```python
from build123d import *

# Parameters (mm, degrees)
SALIENTE_EXTRUIR1_DEPTH = 4
CROQUIS2_R              = 3
CORTAR_EXTRUIR1_DEPTH   = 4
CROQUIS3_R              = 3
CORTAR_EXTRUIR2_DEPTH   = 4
CROQUIS4_R              = 3
CORTAR_EXTRUIR3_DEPTH   = 4


with BuildPart() as part:
    # Croquis1 → Saliente-Extruir1 (new body)
    with BuildSketch(Plane(origin=(0, 0, 0), x_dir=(1, 0, 0), z_dir=(0, 1, 0))):
        Polygon((-82, -35), (-82, -50), (82, -50), (82, -35), (106, -35), (106, 35), (82, 35), (82, 50), (-82, 50), (-82, 35), (-106, 35), (-106, -35), align=None)
    extrude(amount=SALIENTE_EXTRUIR1_DEPTH)

    # Croquis2 → Cortar-Extruir1 (cut)
    with BuildSketch(Plane(origin=(0, 4, 0), x_dir=(1, 0, 0), z_dir=(0, 1, 0))):
        with Locations(Location((-96, 0, 0), (0, 0, 270))):
            Circle(CROQUIS2_R)
        with Locations(Location((-96, 15, 0), (0, 0, 270))):
            Circle(CROQUIS2_R)
        with Locations(Location((-96, -15, 0), (0, 0, 270))):
            Circle(CROQUIS2_R)
    extrude(amount=-CORTAR_EXTRUIR1_DEPTH, mode=Mode.SUBTRACT)

    # Croquis3 → Cortar-Extruir2 (cut)
    with BuildSketch(Plane(origin=(0, 4, 0), x_dir=(1, 0, 0), z_dir=(0, 1, 0))):
        with Locations(Location((96, 15, 0), (0, 0, 270))):
            Circle(CROQUIS3_R)
        with Locations(Location((96, -15, 0), (0, 0, 270))):
            Circle(CROQUIS3_R)
        with Locations(Location((96, 0, 0), (0, 0, 270))):
            Circle(CROQUIS3_R)
    extrude(amount=-CORTAR_EXTRUIR2_DEPTH, mode=Mode.SUBTRACT)

    # Croquis4 → Cortar-Extruir3 (cut)
    with BuildSketch(Plane(origin=(0, 4, 0), x_dir=(1, 0, 0), z_dir=(0, 1, 0))):
        with Locations(Location((0, 25, 0), (0, 0, 270))):
            Circle(CROQUIS4_R)
        with Locations(Location((50, 0, 0), (0, 0, 270))):
            Circle(CROQUIS4_R)
        with Locations(Location((0, -25, 0), (0, 0, 270))):
            Circle(CROQUIS4_R)
        with Locations(Location((-50, 0, 0), (0, 0, 270))):
            Circle(CROQUIS4_R)
        with Locations(Location((0, 0, 0), (0, 0, 270))):
            Circle(CROQUIS4_R)
    extrude(amount=-CORTAR_EXTRUIR3_DEPTH, mode=Mode.SUBTRACT)


solid = part.part
```
CAD build for the part. Positions are in the model's coordinates, mm. A direction names the side the tool comes from. Coordinates: 2 decimals unless noted, no trailing zeros. Write each loop counter-clockwise with the first axis right and the second up, starting at its lowest first coordinate (ties: lowest second). Pieces come first, ordered by that corner, then holes. Notation, with made-up numbers: (-17, 67) -> (12, 67) arc R18 cw to (12, 101) -> close; hole circle Ø8 at (-1, 23.5). An arc over 180 degrees is marked (long way). Use CSV: the item, a comma, the result in double quotes. Start each with the question number.
Item 1: Drop flat-ended pins along their axis: P1, Ø7, axis at x = -50, z = 0, coming from the +Y side; P2, Ø1.2, axis at x = -97, y = 1.5, coming from the +Z side; P3, Ø1.2, axis at y = 3, z = -39, coming from the +X side; P4, Ø1.5, axis at y = 0.5, z = -38, coming from the -X side. Give the stop position or say it passes through.
Item 2: Wall check: probe 1 along X at (y, z) = (1.95, 0); probe 2 along X at (y, z) = (1.6, -15); probe 3 along Z at (x, y) = (-90, 0.3). Give the ranges that are in metal, low to high.
Item 3: Band-saw the part on A-A, the plane x = -50. Write the cut outline in (y, z).
Item 4: Tool access for faces 1 (the flat face through (82, 2, -42)), 2 (the flat face through (-82, 2, -43)), 3 (the flat face through (-94, 2, 35)), 4 (the flat face through (94, 2, 35)): list every direction of +Z, -Z, +X, -X, +Y, -Y with a clear straight run to the whole face (end or side of a thin tool).
Item 5: Band-saw the part on C-C, the plane y = 1. Give the number of separate pieces and of enclosed holes in the cut face, plus the area to 3 significant figures.
Item 6: Band-saw the part on B-B, the plane z = -15. Write the cut outline in (x, y), plus the area to 3 significant figures.
Item 7: Band-saw the part on D-D, the plane z = 25. Write the cut outline in (x, y).
Item 8: Two-plate mould, pull along X, no slides. Class faces 5 (the flat face through (-82, 2, 42)), 6 (the flat face through (-1, 4, 10)), 7 (the cylindrical face through (93.07, 2.03, -15.65)), 8 (the cylindrical face through (93.07, 2.03, -0.65)): +X half, -X half, draft (parallel to the pull), parting line (faces both ways), or undercut.
Response values:
1,P1,"stops at y = 4"
1,P2,"stops at z = 35"
1,P3,"stops at x = 82"
1,P4,"stops at x = -82"
2,probe 1,"x = -106 to -99, -93 to -53, -47 to -3, 3 to 47, 53 to 93, 99 to 106"
2,probe 2,"x = -106 to -99, -93 to 93, 99 to 106"
2,probe 3,"z = -35 to 35"
3,outline,"(0, -50) -> (4, -50) -> (4, -3) -> (0, -3) -> close; (0, 3) -> (4, 3) -> (4, 50) -> (0, 50) -> close"
4,face 1,"-Z, +X, +Y, -Y"
4,face 2,"-Z, -X, +Y, -Y"
4,face 3,"+Z, -X, +Y, -Y"
4,face 4,"+Z, +X, +Y, -Y"
5,separate pieces,"1"
5,enclosed holes,"11"
5,area,"19,400 mm2"
6,outline,"(-106, 0) -> (-99, 0) -> (-99, 4) -> (-106, 4) -> close; (-93, 0) -> (93, 0) -> (93, 4) -> (-93, 4) -> close; (99, 0) -> (106, 0) -> (106, 4) -> (99, 4) -> close"
6,area,"800 mm2"
7,outline,"(-106, 0) -> (-3, 0) -> (-3, 4) -> (-106, 4) -> close; (3, 0) -> (106, 0) -> (106, 4) -> (3, 4) -> close"
8,face 5,"-X half"
8,face 6,"draft"
8,face 7,"undercut"
8,face 8,"undercut"
